The model under review builds one solid part; all positions refer to its coordinate system, in mm. Give positions to 0.01 mm unless a question says otherwise; leave off trailing zeros. Order: outer loops, then holes, each group sorted by start corner. A loop starts at its lowest first (then second) coordinate and runs counter-clockwise, first axis right, second up. Notation, with made-up numbers: (86, -38) - (111, -38) arc R22 cw to (111, -2) - close; hole circle Ø3 at (70, -17). An arc over 180 degrees is marked (long way). Put each result on its own line as item: value.
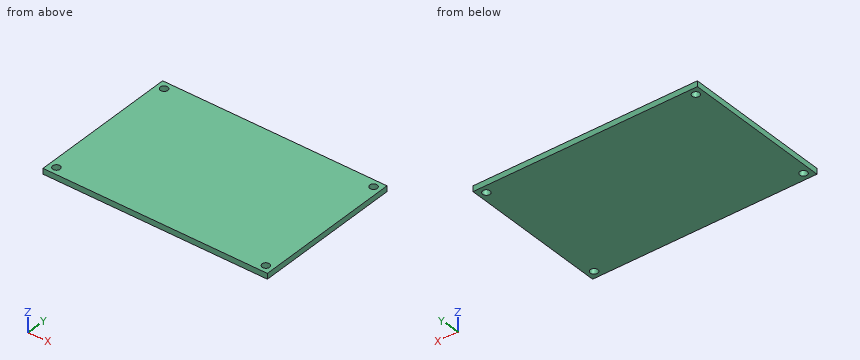
```python
from build123d import *

# Parameters (mm, degrees)
F1_W     = 60
F1_H     = 40
F2_DEPTH = 1.5
F3_R     = 1
F4_DEPTH = 1.5


with BuildPart() as f2:
    # F1 (on Top) → F2 (new body)
    with BuildSketch(Plane.XY):
        Rectangle(F1_W, F1_H)
    extrude(amount=F2_DEPTH)

    # F3 (on face) → F4 (cut, through all)
    with BuildSketch(Plane.XY):
        with Locations((-28, 18)):
            Circle(F3_R)
        with Locations((28, 18)):
            Circle(F3_R)
        with Locations((28, -18)):
            Circle(F3_R)
        with Locations((-28, -18)):
            Circle(F3_R)
    extrude(amount=F4_DEPTH, mode=Mode.SUBTRACT)


solid = f2.part
```
(1) Take a section at B-B, the plane y = -18. Write out the cut boundary in (x, z), then the cut area to 3 significant figures.
The answers:
outline: (-30, 0) - (-29, 0) - (-29, 1.5) - (-30, 1.5) - close; (-27, 0) - (27, 0) - (27, 1.5) - (-27, 1.5) - close; (29, 0) - (30, 0) - (30, 1.5) - (29, 1.5) - close
area: 84.0 mm^2
(2) Wall thickness on L1, parallel to Y at x = 28, z = 0.8: over which ranges is the line inside the solid? List them lowest first.
The answers:
L1: -20 to -19, -17 to 17, 19 to 20
(3) Clearance check with a flat-ended pin moving along its axis: pin 1 Ø1.2 at (x, y) = (28, 18) entering from -Z. State where the tip first meets the part, or that it passes through.
The answers:
pin 1: through
(4) Take a section at A-A, the plane x = -28. Write out the cut boundary in (y, z).
The answers:
outline: (-20, 0) - (-19, 0) - (-19, 1.5) - (-20, 1.5) - close; (-17, 0) - (17, 0) - (17, 1.5) - (-17, 1.5) - close; (19, 0) - (20, 0) - (20, 1.5) - (19, 1.5) - close
